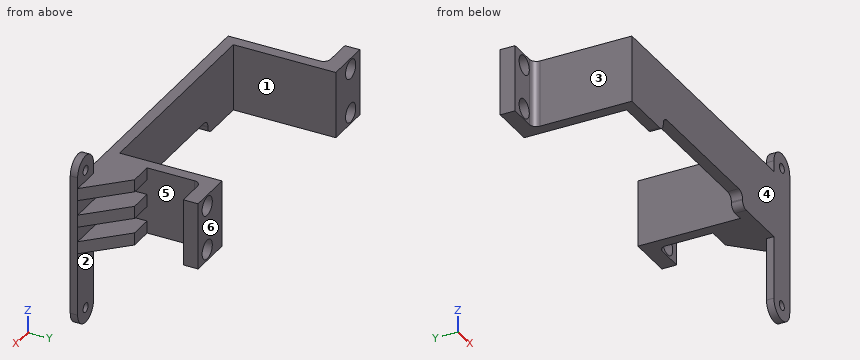
```python
from build123d import *

# Parameters (mm, degrees)
BOSS_EXTRUDE1_DEPTH = 22.86
SKETCH2_R           = 1.5875
BOSS_EXTRUDE2_DEPTH = 2.54
SKETCH4_W           = 15.367
SKETCH4_H           = 22.86
SKETCH4_R           = 3.2639
BOSS_EXTRUDE3_DEPTH = 5.08
SKETCH5_W           = 20.701
SKETCH5_H           = 4.233333333
SKETCH5_H_2         = 4.233333334
BOSS_EXTRUDE4_DEPTH = 12.7
CHAMFER1_SIZE       = 12.7
FILLET1_R           = 2.38
SKETCH6_W           = 50.8
SKETCH6_H           = 5.08
CUT_EXTRUDE1_DEPTH  = 110.560976655
FILLET2_R           = 2.38


with BuildPart() as part:
    # Sketch1 → Boss-Extrude1 (new body)
    with BuildSketch(Plane.XY):
        Polygon((-3.81, 35.052), (0, 35.052), (0, 0), (72.898, 0), (72.898, 35.052), (76.708, 35.052), (76.708, -3.81), (-3.81, -3.81), align=None)
    extrude(amount=BOSS_EXTRUDE1_DEPTH)

    # Sketch2 → Boss-Extrude2 (add)
    with BuildSketch(Plane.XZ.offset(3.81)):
        with BuildLine():
            ThreePointArc((97.409, 26.6192), (92.329, 31.6992), (87.249, 26.6192))
            Line((87.249, 26.6192), (87.249, 22.86))
            Line((87.249, 22.86), (76.708, 22.86))
            Line((76.708, 22.86), (76.708, 0))
            Line((76.708, 0), (87.249, 0))
            Line((87.249, 0), (87.249, -21.5392))
            ThreePointArc((87.249, -21.5392), (92.329, -26.6192), (97.409, -21.5392))
            Line((97.409, -21.5392), (97.409, 26.6192))
        make_face()
        with Locations((92.329, -21.5392)):
            Circle(SKETCH2_R, mode=Mode.SUBTRACT)
        with Locations((92.329, 26.6192)):
            Circle(SKETCH2_R, mode=Mode.SUBTRACT)
    extrude(amount=-BOSS_EXTRUDE2_DEPTH)

    # Sketch4 → Boss-Extrude3 (add)
    with BuildSketch(Plane(origin=(0, 35.052, 0), x_dir=(1, 0, 0), z_dir=(0, 1, 0))):
        with Locations((-7.6835, -11.43)):
            Rectangle(SKETCH4_W, SKETCH4_H)
        with Locations(Location((-9.525, -3.81, 0), (0, 0, 270))):
            Circle(SKETCH4_R, mode=Mode.SUBTRACT)
        with Locations(Location((-9.525, -19.05, 0), (0, 0, 270))):
            Circle(SKETCH4_R, mode=Mode.SUBTRACT)
    boss_extrude3 = extrude(amount=-BOSS_EXTRUDE3_DEPTH)

    # Mirror1: Boss-Extrude3 across plane
    add(boss_extrude3.mirror(Plane(origin=(36.449, 0, 0), x_dir=(0, 0, 1), z_dir=(1, 0, 0))))

    # Sketch5 → Boss-Extrude4 (add)
    with BuildSketch(Plane(origin=(0, -1.27, 0), x_dir=(1, 0, 0), z_dir=(0, 1, 0))):
        with Locations((87.0585, -2.116666667)):
            Rectangle(SKETCH5_W, SKETCH5_H)
        with Locations((87.0585, -20.743333334)):
            Rectangle(SKETCH5_W, SKETCH5_H)
        with Locations((87.0585, -11.43)):
            Rectangle(SKETCH5_W, SKETCH5_H_2)
    extrude(amount=BOSS_EXTRUDE4_DEPTH)

    # Chamfer1
    chamfer1_edges = [part.edges().sort_by_distance(p)[0] for p in [
        (97.409, 11.43, 20.743333333),
        (97.409, 11.43, 11.43),
        (97.409, 11.43, 2.116666667),
    ]]
    chamfer(chamfer1_edges, length=CHAMFER1_SIZE)

    # Fillet1
    fillet1_edges = [part.edges().sort_by_distance(p)[0] for p in [
        (-3.81, 29.972, 11.43),
        (76.708, 29.972, 11.43),
    ]]
    fillet(fillet1_edges, radius=FILLET1_R)

    # Sketch6 → Cut-Extrude1 (cut, through all)
    with BuildSketch(Plane.XZ.offset(3.81)):
        with Locations((41.7195, 2.54)):
            Rectangle(SKETCH6_W, SKETCH6_H)
    extrude(amount=-CUT_EXTRUDE1_DEPTH, mode=Mode.SUBTRACT)

    # Fillet2
    fillet2_edges = [part.edges().sort_by_distance(p)[0] for p in [
        (16.3195, -1.905, 0),
        (67.1195, -1.905, 0),
        (16.3195, -1.905, 5.08),
        (67.1195, -1.905, 5.08),
    ]]
    fillet(fillet2_edges, radius=FILLET2_R)


solid = part.part
```
Here's how the part is built. I have some questions about the finished solid (model axes, mm). Face numbers are marked on the shaded views. A direction names the side the tool comes from. Round coordinates to 2 decimals unless told otherwise and drop trailing zeros. Write each loop counter-clockwise with the first axis right and the second up, starting at its lowest first coordinate (ties: lowest second). Pieces come first, ordered by that corner, then holes.
Q1. Please list where these lines run through material, in increasing order: probe 1 along X at (y, z) = (33, 19) (3 decimals); probe 2 along X at (y, z) = (32, 3) (3 decimals); probe 3 along X at (y, z) = (31, 12) (3 decimals).
Q2. Which directions (+Z, -Z, +X, -X, +Y, -Y) give clear straight access to the entire face, cutting with the end or side of a thin tool? Please do the marked faces 1, 2, 3 and 4.
Q3. Will these pins go through, and if not, where does the flat tip stop? P1, Ø8.5, axis at x = -9.525, z = 3.81, coming from the +Y side; P2, Ø9.5, axis at x = 90.5, z = 29, coming from the +Y side; P3, Ø7, axis at y = 25, z = 14.5, coming from the +X side; P4, Ø8, axis at x = 4.5, y = 8.5, coming from the -Z side.
Q4. If we mould it in two halves opening along Z, with no side actions, what happens to the marked faces 5 and 6? For each: +Z half, -Z half, draft (parallel to the pull), parting line (faces both ways), or undercut.
Q5. If we section it at A-A on y = 12.5: Write out the boundary of the cut face in (x, z).
Q6. If we section it at B-B on z = -5.5: Write out the boundary of the cut face in (x, y).
Q7. If we section it at C-C on y = 4.5: Write out the boundary of the cut face in (x, z).
Answer below:
1. probe 1: x = -15.367 to -12.789, -6.261 to 0, 72.898 to 79.159, 85.687 to 88.265
1. probe 2: x = -15.367 to -12.687, -6.363 to 0, 72.898 to 79.261, 85.585 to 88.265
1. probe 3: x = -15.367 to 0, 72.898 to 88.265
2. face 1: +Z, -Z, +Y
2. face 2: -Z, +X, -X, +Y
2. face 3: +Z, -Z, -X, -Y
2. face 4: +Z, -Z, +X, -X, -Y
3. P1: stops at y = 35.05
3. P2: stops at y = -1.27
3. P3: stops at x = 76.89
3. P4: passes through
4. face 5: undercut
4. face 6: draft
5. outline: (-3.81, 0) - (0, 0) - (0, 22.86) - (-3.81, 22.86) - close; (72.9, 0) - (76.71, 0) - (76.71, 22.86) - (72.9, 22.86) - close
6. outline: (87.25, -3.81) - (97.41, -3.81) - (97.41, -1.27) - (87.25, -1.27) - close
7. outline: (-3.81, 0) - (0, 0) - (0, 22.86) - (-3.81, 22.86) - close; (72.9, 0) - (91.64, 0) - (91.64, 4.23) - (76.71, 4.23) - (76.71, 9.31) - (91.64, 9.31) - (91.64, 13.55) - (76.71, 13.55) - (76.71, 18.63) - (91.64, 18.63) - (91.64, 22.86) - (72.9, 22.86) - close
